Source: three-view drawing plus pictorial views. Frame: mm from the lowest corner of the part. Give positions to 0.01 mm unless a question says otherwise; leave off trailing zeros. Loops run counter-clockwise (first coordinate to the right, second up) from the corner with the lowest first, then second, coordinate; pieces in that order, holes last. Notation, with made-up numbers: M -25.75,-33.75 L 14.25,-33.75 A18 cw 14.25,-1.75 Z; hole C 10.5,23 d4. An arc over 180 degrees is marked long. One line per item, written item: value. Start each with the question number.
(1) Ray query, line 1 along Z through (x, y) = (111, 43); line 2 along Z through (x, y) = (131.5, 4) (1 decimal). Return the intervals inside material, ascending. Write a range as from..to.
(2) Section A-A on y = 31. Output: boundary loops of the cut face in (x, z) (1 decimal), plus the area to 3 significant figures.
(3) Pin query (flat end, axial travel): P1, Ø12, axis at x = 114.5, y = 35, coming from the +Z side (1 decimal); P2, Ø1, axis at y = 5, z = 18, coming from the -X side (1 decimal). Return the tip coordinate at first contact, or that it passes through.
(4) Section C-C on z = 24.5. Output: boundary loops of the cut face in (x, y), plus the area to 3 significant figures.
(5) Section B-B on x = 26.5. Output: boundary loops of the cut face in (y, z) (1 decimal).
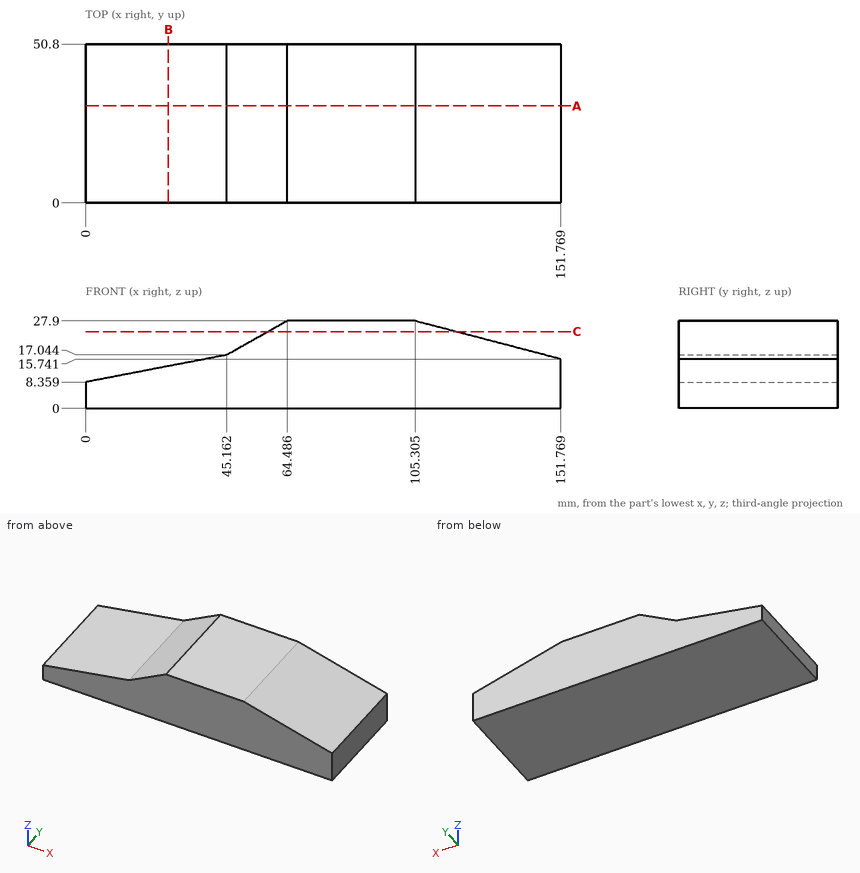
Output values:
1. line 1: z = 0..26.41
1. line 2: z = 0..21
2. outline: M 0,0 L 151.8,0 L 151.8,15.7 L 105.3,27.9 L 64.5,27.9 L 45.2,17 L 0,8.4 Z
2. area: 3,160 mm²
3. P1: stops at z = 27.1
3. P2: stops at x = 46
4. outline: M 58.43,0 L 118.3,0 L 118.3,50.8 L 58.43,50.8 Z
4. area: 3,040 mm²
5. outline: M 0,0 L 50.8,0 L 50.8,13.5 L 0,13.5 Z
